Here's how the part is built. I have some questions about the finished solid (model axes, mm). Face numbers are marked on the shaded views. A direction names the side the tool comes from. Coordinates: 2 decimals unless noted, no trailing zeros. Write each loop counter-clockwise with the first axis right and the second up, starting at its lowest first coordinate (ties: lowest second). Pieces come first, ordered by that corner, then holes. Notation, with made-up numbers: (48, 67) -> (81, 67) arc R21 ccw to (81, 91) -> close; hole circle Ø9 at (-25, 45). An arc over 180 degrees is marked (long way). Use CSV: the item, a comma, the result in double quotes. Start each with the question number.
```python
from build123d import *

# Parameters (mm, degrees)
CHAFL_N1_SIZE                = 0.5
TALADRO_DE_MARGEN_PARA_M41_D = 4.5
TALADRO_DE_MARGEN_PARA_M31_D = 3.2


with BuildPart() as part:
    # Croquis1 → Revolución1 (revolve)
    with BuildSketch(Plane(origin=(0, 0, 0), x_dir=(-1, 0, 0), z_dir=(0, 1, 0)), mode=Mode.PRIVATE) as revoluci_n1_sk:
        Polygon((-42.75, 0), (42.75, 0), (42.75, 3), (30.25, 3), (30.25, 4), (20.25, 4), (20.25, 6), (-30.75, 6), (-30.75, 4), (-42.75, 4), align=None)
    revolve(revoluci_n1_sk.sketch.rotate(Axis((42.75, 0, 0), (-1, 0, 0)), 180), axis=Axis((42.75, 0, 0), (-1, 0, 0)))

    # Chaflán1
    chafl_n1_edges = [part.edges().sort_by_distance(p)[0] for p in [
        (-42.75, 0, 3),
        (42.75, 0, 4),
    ]]
    chamfer(chafl_n1_edges, length=CHAFL_N1_SIZE)

    # Taladro de margen para M41 (through all)
    with Locations(Plane(origin=(0, 10, 0), x_dir=(-1, 0, 0), z_dir=(0, 1, 0))):
        with Locations((11.25, 0), (-0.75, 0)):
            Hole(TALADRO_DE_MARGEN_PARA_M41_D / 2)

    # Taladro de margen para M31 (through all)
    with Locations(Plane(origin=(0, 10, 0), x_dir=(-1, 0, 0), z_dir=(0, 1, 0))):
        with Locations((-24.75, 0)):
            Hole(TALADRO_DE_MARGEN_PARA_M31_D / 2)


solid = part.part
```
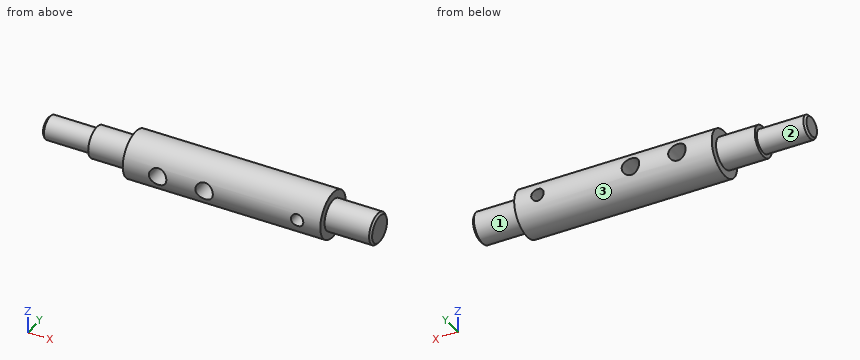
Item 1: I want a section at D-D on x = 24.75. Please give me the cut outline in (y, z).
Item 2: If I drill on line 1 along X through (y, z) = (1.5, 0); line 2 along X through (y, z) = (-4.5, 0.25); line 3 along X through (y, z) = (-3.5, 3), over which ranges is the centre line in solid material (lowest first)?
Item 3: I'm going to push flat-ended pins straight in: pin 1 (4 mm diameter, centred on x = -11.25, z = 0, fed in from -Y); pin 2 (1 mm diameter, centred on x = 8.5, y = 2.5, fed in from +Z); pin 3 (4 mm diameter, centred on x = 33, z = -2.5, fed in from -Y); pin 4 (2 mm diameter, centred on x = 33, z = 1.5, fed in from +Y). Where does each tip first touch, or does it pass through?
Item 4: I want a section at B-B on y = 0. Please give me the cut outline in (x, z), then the cut area to 3 significant figures.
Item 5: I want a section at A-A on z = 0. Count the separate pieces of the cut face and the enclosed holes in it, then the cut area to 3 significant figures.
Item 6: I want a section at C-C on x = -36. Please give me the cut outline in (y, z), then the cut area to 3 significant figures.
Item 7: Which directions (+Z, -Z, +X, -X, +Y, -Y) give clear straight access to the entire face, cutting with the end or side of a thin tool? Please do the marked faces 1, 2 and 3.
Geometry says:
1,outline,"(-5.78, -1.6) arc R6 ccw to (5.78, -1.6) -> close; (-5.78, 1.6) -> (5.78, 1.6) arc R6 ccw to start"
2,line 1,"-42.75 to -13.5, -9 to -1.5, 3 to 23.15, 26.35 to 42.75"
2,line 2,"-20.25 to -13.49, -9.01 to -1.49, 2.99 to 23.17, 26.33 to 30.75"
2,line 3,"-20.25 to 30.75"
3,pin 1,"through"
3,pin 2,"z = 5.66"
3,pin 3,"y = -3.97"
3,pin 4,"y = 3.97"
4,outline,"(-42.75, -2.5) -> (-42.25, -3) -> (-30.25, -3) -> (-30.25, -4) -> (-20.25, -4) -> (-20.25, -6) -> (30.75, -6) -> (30.75, -4) -> (42.25, -4) -> (42.75, -3.5) -> (42.75, 3.5) -> (42.25, 4) -> (30.75, 4) -> (30.75, 6) -> (-20.25, 6) -> (-20.25, 4) -> (-30.25, 4) -> (-30.25, 3) -> (-42.25, 3) -> (-42.75, 2.5) -> close; hole circle Ø4.5 at (-11.25, 0); hole circle Ø4.5 at (0.75, 0); hole circle Ø3.2 at (24.75, 0)"
4,area,"823 mm2"
5,separate pieces,"4"
5,enclosed holes,"0"
5,area,"716 mm2"
6,outline,"circle Ø6 at (0, 0)"
6,area,"28.3 mm2"
7,face 1,"+X"
7,face 2,"-X"
7,face 3,"+X, -X"
